from build123d import *

# Parameters (mm, degrees)
SKETCH_1_W      = 538
SKETCH_1_H      = 50
EXTRUDE_1_DEPTH = 6


with BuildPart() as part:
    # Эскиз1 → Бобышка-Вытянуть1 (new body)
    with BuildSketch(Plane.XY):
        with Locations((95.16967509, -17.799165817)):
            Rectangle(SKETCH_1_W, SKETCH_1_H)
        with BuildLine():
            Line((-25.83032491, -7.799165817), (216.16967509, -7.799165817))
            ThreePointArc((216.16967509, -7.799165817), (218.998102215, -8.970738692), (220.16967509, -11.799165817))
            Line((220.16967509, -11.799165817), (220.16967509, -23.799165817))
            ThreePointArc((220.16967509, -23.799165817), (218.998102215, -26.627592942), (216.16967509, -27.799165817))
            Line((216.16967509, -27.799165817), (-25.83032491, -27.799165817))
            ThreePointArc((-25.83032491, -27.799165817), (-28.658752034, -26.627592942), (-29.83032491, -23.799165817))
            Line((-29.83032491, -23.799165817), (-29.83032491, -11.799165817))
            ThreePointArc((-29.83032491, -11.799165817), (-28.658752034, -8.970738692), (-25.83032491, -7.799165817))
        make_face(mode=Mode.SUBTRACT)
    extrude(amount=EXTRUDE_1_DEPTH)


solid = part.part
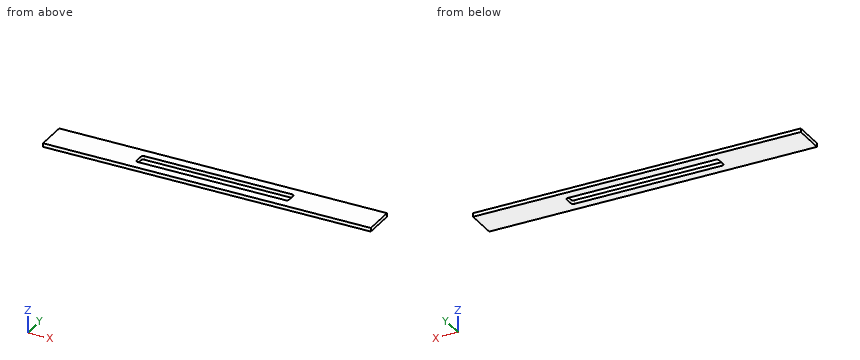
The listing builds one solid part. Answer for the finished solid, in the listing's coordinates (mm). Round coordinates to 2 decimals unless told otherwise and drop trailing zeros. Loops run counter-clockwise (first coordinate to the right, second up) from the corner with the lowest first, then second, coordinate; pieces in that order, holes last. Notation, with made-up numbers: M 70.5,22.25 L 112.5,22.25 A28 cw 112.5,46.25 Z; hole C 14.5,-21 d1. An arc over 180 degrees is marked long. Return JSON: item names as keys, results as strings.
Q1. Find section A-A, the plane z = 3.4. Determine the outline of the cut face in (x, y), plus the area to 3 significant figures.
Results list:
{"outline": "M -173.83,-42.8 L 364.17,-42.8 L 364.17,7.2 L -173.83,7.2 Z; hole M -29.83,-23.8 A4 ccw -25.83,-27.8 L 216.17,-27.8 A4 ccw 220.17,-23.8 L 220.17,-11.8 A4 ccw 216.17,-7.8 L -25.83,-7.8 A4 ccw -29.83,-11.8 Z", "area": "21,900 mm2"}
Q2. Find the intervals of material crossed by line 1 along X through (y, z) = (-22, 3.9); line 2 along Y through (x, z) = (125, 5.35); line 3 along X through (y, z) = (-25.5, 5.4), in increasing order. Write a range as from..to.
Results list:
{"line 1": "x = -173.83..-29.83, 220.17..364.17", "line 2": "y = -42.8..-27.8, -7.8..7.2", "line 3": "x = -173.83..-29.45, 219.79..364.17"}
Q3. Find section B-B, the plane x = 188. Determine the outline of the cut face in (y, z), plus the area to 3 significant figures.
Results list:
{"outline": "M -42.8,0 L -27.8,0 L -27.8,6 L -42.8,6 Z; M -7.8,0 L 7.2,0 L 7.2,6 L -7.8,6 Z", "area": "180 mm2"}
